Design review of the part built by this model. Coordinates are the model's own, in mm. A direction names the side the tool comes from. Coordinates: 2 decimals unless noted, no trailing zeros. Write each loop counter-clockwise with the first axis right and the second up, starting at its lowest first coordinate (ties: lowest second). Pieces come first, ordered by that corner, then holes. Notation, with made-up numbers: M 6,-13 L 31,-13 A17 cw 31,4 Z; hole C -14,-1.5 d9. An arc over 180 degrees is marked long. Write item = value, one per line.
```python
from build123d import *

# Parameters (mm, degrees)
SKETCH1_W           = 300
SKETCH1_H           = 200
BOSS_EXTRUDE1_DEPTH = 3.175
SKETCH6_R           = 4
CUT_EXTRUDE2_DEPTH  = 4.175
FILLET1_R           = 6.35
SKETCH2_R           = 1.5
CUT_EXTRUDE1_DEPTH  = 4.175
SKETCH16_R          = 1.89865
M5_THROUGH_DEPTH    = 4.175
SKETCH9_R           = 1.75
SKETCH9_R_2         = 1.89865
CUT_EXTRUDE3_DEPTH  = 4.175
SKETCH10_R          = 1.89865
SKETCH10_R_2        = 1.9939
CUT_EXTRUDE5_DEPTH  = 4.175
SKETCH17_R          = 1.75
M3_THROUGH_DEPTH    = 4.175
FILLET2_R           = 6.35


with BuildPart() as part:
    # Sketch1 → Boss-Extrude1 (new body)
    with BuildSketch(Plane(origin=(0, 0, 0), x_dir=(1, 0, 0), z_dir=(0, 1, 0))):
        with Locations((150, 100)):
            Rectangle(SKETCH1_W, SKETCH1_H)
    extrude(amount=BOSS_EXTRUDE1_DEPTH)

    # Sketch6 → Cut-Extrude2 (cut, through all)
    with BuildSketch(Plane(origin=(0, 3.175, 0), x_dir=(1, 0, 0), z_dir=(0, 1, 0))):
        with Locations((150, 118.651)):
            Circle(SKETCH6_R)
    extrude(amount=-CUT_EXTRUDE2_DEPTH, mode=Mode.SUBTRACT)

    # Fillet1
    fillet1_edges = [part.edges().sort_by_distance(p)[0] for p in [
        (0, 1.5875, -200),
        (300, 1.5875, -200),
        (300, 1.5875, 0),
        (0, 1.5875, 0),
    ]]
    fillet(fillet1_edges, radius=FILLET1_R)

    # Sketch2 → Cut-Extrude1 (cut, through all)
    with BuildSketch(Plane(origin=(0, 3.175, 0), x_dir=(1, 0, 0), z_dir=(0, 1, 0))):
        with Locations((6.35, 174.6)):
            Circle(SKETCH2_R)
        with Locations((6.35, 49.9999)):
            Circle(SKETCH2_R)
        with Locations((249.2, 75.3999)):
            Circle(SKETCH2_R)
        with Locations((50.8, 75.3999)):
            Circle(SKETCH2_R)
        with Locations((293.65, 49.9999)):
            Circle(SKETCH2_R)
        with Locations((50.8, 24.5999)):
            Circle(SKETCH2_R)
        with Locations((249.2, 24.5999)):
            Circle(SKETCH2_R)
        with Locations((25.4, 193.65)):
            Circle(SKETCH2_R)
        with Locations((274.6, 193.65)):
            Circle(SKETCH2_R)
        with Locations((293.65, 174.6)):
            Circle(SKETCH2_R)
    extrude(amount=-CUT_EXTRUDE1_DEPTH, mode=Mode.SUBTRACT)

    # Sketch16 → M5_through (cut, through all)
    with BuildSketch(Plane(origin=(0, 3.175, -5.8), x_dir=(1, 0, 0), z_dir=(0, -1, 0))):
        with Locations((118.25, -18.651)):
            Circle(SKETCH16_R)
        with Locations((139.416666667, -0.55096)):
            Circle(SKETCH16_R)
        with Locations((160.583333333, -0.55096)):
            Circle(SKETCH16_R)
        with Locations((181.75, -18.651)):
            Circle(SKETCH16_R)
    extrude(amount=M5_THROUGH_DEPTH, mode=Mode.SUBTRACT)

    # Sketch9 → Cut-Extrude3 (cut, through all)
    with BuildSketch(Plane(origin=(0, 3.175, 0), x_dir=(-1, 0, 0), z_dir=(0, 1, 0))):
        with Locations((-118.25, -15.40098)):
            Circle(SKETCH9_R)
        with Locations((-150, -6.35096)):
            Circle(SKETCH9_R)
        with Locations((-181.75, -15.40098)):
            Circle(SKETCH9_R)
        with Locations((-160.583333333, -6.35096)):
            Circle(SKETCH9_R_2)
    extrude(amount=-CUT_EXTRUDE3_DEPTH, mode=Mode.SUBTRACT)

    # Sketch10 → Cut-Extrude5 (cut, through all)
    with BuildSketch(Plane(origin=(0, 3.175, 0), x_dir=(1, 0, 0), z_dir=(0, 1, 0))):
        with Locations((160, 135.971508076)):
            Circle(SKETCH10_R)
        with Locations((150, 138.651)):
            Circle(SKETCH10_R_2)
        with Locations((167.320508076, 128.651)):
            Circle(SKETCH10_R_2)
        with Locations((167.320508076, 108.651)):
            Circle(SKETCH10_R_2)
        with Locations((150, 98.651)):
            Circle(SKETCH10_R_2)
        with Locations((132.679491924, 108.651)):
            Circle(SKETCH10_R_2)
        with Locations((132.679491924, 128.651)):
            Circle(SKETCH10_R_2)
        with Locations((170, 118.651)):
            Circle(SKETCH10_R)
        with Locations((160, 101.330491924)):
            Circle(SKETCH10_R)
        with Locations((140, 101.330491924)):
            Circle(SKETCH10_R)
        with Locations((130, 118.651)):
            Circle(SKETCH10_R)
        with Locations((140, 135.971508076)):
            Circle(SKETCH10_R)
        with BuildLine():
            Line((124.6, 75.583146559), (124.6, 37.151))
            Line((124.6, 37.151), (92.85, 37.151))
            Line((92.85, 37.151), (92.85, 0))
            Line((92.85, 0), (0, 0))
            Line((0, 0), (0, 200))
            Line((0, 200), (300, 200))
            Line((300, 200), (300, 0))
            Line((300, 0), (207.15, 0))
            Line((207.15, 0), (207.15, 37.151))
            Line((207.15, 37.151), (175.4, 37.151))
            Line((175.4, 37.151), (175.4, 75.583146559))
            ThreePointArc((175.4, 75.583146559), (150, 168.651), (124.6, 75.583146559))
        make_face()
    extrude(amount=-CUT_EXTRUDE5_DEPTH, mode=Mode.SUBTRACT)

    # Sketch17 → M3-through (cut, through all)
    with BuildSketch(Plane(origin=(0, 3.175, 0), x_dir=(1, 0, 0), z_dir=(0, 1, 0))):
        with Locations((185, 118.651)):
            Circle(SKETCH17_R)
        with Locations((167.5, 88.340110868)):
            Circle(SKETCH17_R)
        with Locations((132.5, 88.340110868)):
            Circle(SKETCH17_R)
        with Locations((115, 118.651)):
            Circle(SKETCH17_R)
        with Locations((132.5, 148.961889132)):
            Circle(SKETCH17_R)
        with Locations((167.5, 148.961889132)):
            Circle(SKETCH17_R)
    extrude(amount=-M3_THROUGH_DEPTH, mode=Mode.SUBTRACT)

    # Fillet2
    fillet2_edges = [part.edges().sort_by_distance(p)[0] for p in [
        (175.4, 1.5875, -75.583146559),
        (124.6, 1.5875, -75.583146559),
        (124.6, 1.5875, -37.151),
        (92.85, 1.5875, -37.151),
        (92.85, 1.5875, 0),
        (207.15, 1.5875, 0),
        (207.15, 1.5875, -37.151),
        (175.4, 1.5875, -37.151),
    ]]
    fillet(fillet2_edges, radius=FILLET2_R)


solid = part.part
```
Q1. Consider section B-B, the plane z = -60.5. State the section outline as (x, y) points (3 decimals).
Check result:
outline = M 124.6,0 L 175.4,0 L 175.4,3.175 L 124.6,3.175 Z
Q2. The part is to be moulded in two halves that separate along Z. For faces 1 (the flat face through (149, 0, -86)), 2 (the flat face through (149, 2, 0)), 3 (the cylindrical face through (116.58, 1.61, -14.88)), say which applies: +Z half, -Z half, draft (parallel to the pull), parting line (faces both ways), or undercut.
Check result:
face_1 = draft
face_2 = +Z half
face_3 = undercut
Q3. For P1, Ø4, axis at x = 132.5, z = -88.34, coming from the +Y side (3 decimals); P2, Ø1.5, axis at y = 1.5, z = -133, coming from the -X side; P3, Ø3, axis at x = 132.5, z = -148.96, coming from the +Y side, all flat-tipped, find the tip position at first contact; note any pin that passes through.
Check result:
P1 = 3.175
P2 = 101.88
P3 = through
Q4. Wall thickness on line 1 (Z direction, x = 150, y = 0.9); line 2 (X direction, y = 2.15, z = -54.5); line 3 (X direction, y = 2.7, z = -24): over which ranges is each line inside the solid? List them lowest first.
Check result:
line_1 = -168.65 to -140.64, -136.66 to -122.65, -114.65 to -100.64, -96.66 to -8.1, -4.6 to 0
line_2 = 124.6 to 175.4
line_3 = 92.85 to 116.41, 120.09 to 179.91, 183.59 to 207.15
Q5. Consider section A-A, the plane x = 150. State the section outline as (y, z) points (3 decimals), and give its area (3 significant figures).
Check result:
outline = M 0,-168.651 L 3.175,-168.651 L 3.175,-140.645 L 0,-140.645 Z; M 0,-136.657 L 3.175,-136.657 L 3.175,-122.651 L 0,-122.651 Z; M 0,-114.651 L 3.175,-114.651 L 3.175,-100.645 L 0,-100.645 Z; M 0,-96.657 L 3.175,-96.657 L 3.175,-8.101 L 0,-8.101 Z; M 0,-4.601 L 3.175,-4.601 L 3.175,0 L 0,0 Z
area = 474 mm²
Q6. Consider section C-C, the plane y = 1.75. State how many separate pieces and enclosed holes the cut face has, and give its area (3 significant figures).
Check result:
separate_pieces = 1
enclosed_holes = 26
area = 13,500 mm²
Q7. Machinability: for faces 4 (the flat face through (124.6, 2, -58)), 5 (the flat face through (175.4, 2, -58)), 6 (the cylindrical face through (148.33, 1.61, -5.83)), which of the approach directions +Z, -Z, +X, -X, +Y, -Y give a long, thin tool a straight path to every point of the face, cutting with its end or side? Answer none if there is none.
Check result:
face_4 = -X, +Y, -Y
face_5 = +X, +Y, -Y
face_6 = +Y, -Y
